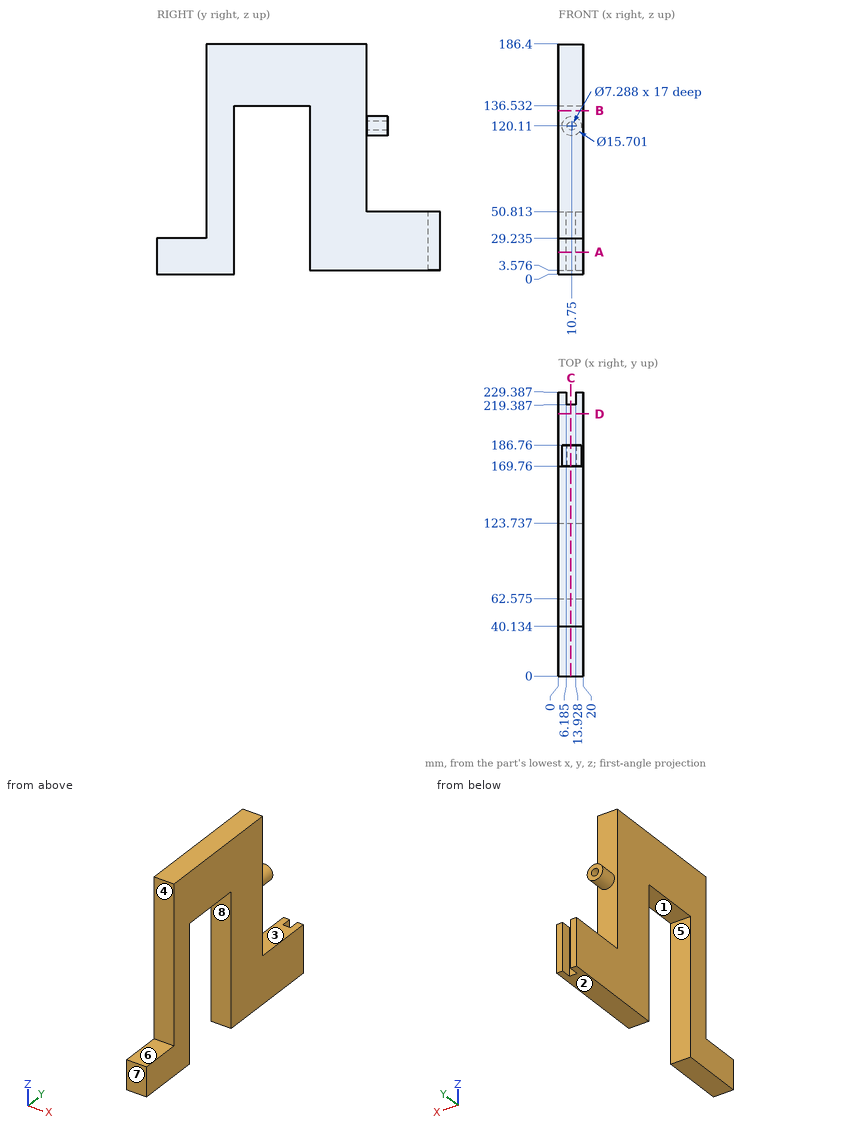
Could you check a few things on this drawing? It's one solid part, dimensions in mm from its lowest x, y, z. A direction names the side the tool comes from. Round coordinates to 2 decimals unless told otherwise and drop trailing zeros. Loops run counter-clockwise (first coordinate to the right, second up) from the corner with the lowest first, then second, coordinate; pieces in that order, holes last. Notation, with made-up numbers: (68.25, 13.25) -> (113.25, 13.25) arc R8 ccw to (113.25, 22.25) -> close; hole circle Ø1 at (-5.5, -37.75). An arc over 180 degrees is marked (long way). One line per item, written item: value. Start each with the question number.
1. If we mould it in two halves opening along Y, with no side actions, what happens to the marked faces 5, 6, 7 and 8? For each: pulls with the +Y half, pulls with the -Y half, needs draft (parallel to the pull), parting line crosses it, or undercut.
2. For pin 1 (6 mm diameter, centred on x = 7.5, y = 98, fed in from -Z); pin 2 (10 mm diameter, centred on x = 7.5, z = 101, fed in from +Y); pin 3 (10 mm diameter, centred on x = 9, y = 199.5, fed in from +Z), each with a flat end and sliding along its axis, tell me the tip position at first contact or that it passes through.
3. If we section it at C-C, the plane x = 10: Write out the boundary of the cut face in (y, z) (1 decimal).
4. If we section it at A-A, the plane z = 18: Write out the boundary of the cut face in (x, y) (1 decimal).
5. For the marked faces 1, 2, 3 and 4, which set-ups out of +Z, -Z, +X, -X, +Y, -Y let a thin tool reach every point of the face, with its end or its side?
6. If we section it at D-D, the plane y = 212: Write out the boundary of the cut face in (x, z).
7. If we section it at B-B, the plane z = 132.5: Write out the boundary of the cut face in (x, y) (1 decimal).
8. If I drill on probe 1 along Y at (x, z) = (1.25, 37.5) (1 decimal); probe 2 along Y at (x, z) = (13.5, 84.5) (1 decimal); probe 3 along Z at (x, y) = (12, 181.5) (1 decimal), over which ranges is the centre line in solid material (lowest first)?
Calculated:
1. face 5: undercut
1. face 6: needs draft
1. face 7: pulls with the -Y half
1. face 8: undercut
2. pin 1: stops at z = 136.53
2. pin 2: stops at y = 169.76
2. pin 3: stops at z = 50.81
3. outline: (0, 0) -> (62.6, 0) -> (62.6, 136.5) -> (123.7, 136.5) -> (123.7, 3.6) -> (219.4, 3.6) -> (219.4, 50.8) -> (169.8, 50.8) -> (169.8, 112.3) -> (186.8, 112.3) -> (186.8, 116.5) -> (169.8, 116.5) -> (169.8, 123.7) -> (186.8, 123.7) -> (186.8, 127.9) -> (169.8, 127.9) -> (169.8, 186.4) -> (40.1, 186.4) -> (40.1, 29.2) -> (0, 29.2) -> close
4. outline: (0, 0) -> (20, 0) -> (20, 62.6) -> (0, 62.6) -> close; (0, 123.7) -> (20, 123.7) -> (20, 229.4) -> (13.9, 229.4) -> (13.9, 219.4) -> (6.2, 219.4) -> (6.2, 229.4) -> (0, 229.4) -> close
5. face 1: -Z, +X, -X
5. face 2: -Z, +X, -X, +Y
5. face 3: +X, -X, +Y
5. face 4: +Z, +X, -X, -Y
6. outline: (0, 3.58) -> (20, 3.58) -> (20, 50.81) -> (0, 50.81) -> close
7. outline: (0, 40.1) -> (20, 40.1) -> (20, 62.6) -> (0, 62.6) -> close; (0, 123.7) -> (20, 123.7) -> (20, 169.8) -> (0, 169.8) -> close
8. probe 1: y = 40.1 to 62.6, 123.7 to 229.4
8. probe 2: y = 40.1 to 62.6, 123.7 to 169.8
8. probe 3: z = 3.6 to 50.8, 112.4 to 116.7, 123.5 to 127.9
